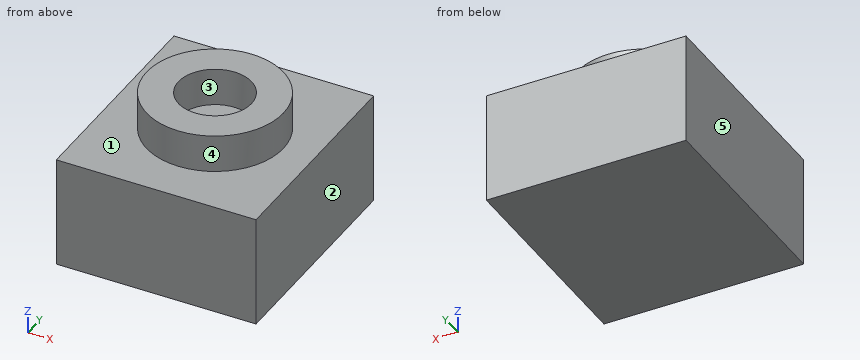
from build123d import *

# Parameters (mm, degrees)
ESQUISSE1_W        = 10.6
ESQUISSE1_H        = 11.7
BOSS_EXTRU_1_DEPTH = 5.9
ESQUISSE2_R        = 3.633546232
ESQUISSE2_R_2      = 1.941835626
BOSS_EXTRU_2_DEPTH = 2


with BuildPart() as part:
    # Esquisse1 → Boss.-Extru.1 (new body)
    with BuildSketch(Plane.XY):
        Rectangle(ESQUISSE1_W, ESQUISSE1_H)
    extrude(amount=BOSS_EXTRU_1_DEPTH)

    # Esquisse2 → Boss.-Extru.2 (add)
    with BuildSketch(Plane.XY.offset(5.9)):
        Circle(ESQUISSE2_R)
        Circle(ESQUISSE2_R_2, mode=Mode.SUBTRACT)
    extrude(amount=BOSS_EXTRU_2_DEPTH)


solid = part.part
Verification items for the finished model (mm, model axes). Face numbers are marked on the shaded views. A direction names the side the tool comes from. Round coordinates to 2 decimals unless told otherwise and drop trailing zeros. Loops run counter-clockwise (first coordinate to the right, second up) from the corner with the lowest first, then second, coordinate; pieces in that order, holes last. Notation, with made-up numbers: (78, -16) - (107, -16) arc R18 ccw to (107, 11) - close; hole circle Ø11 at (2, 32.25). An arc over 180 degrees is marked (long way). Use one line per item in the form item = value.
1. Draft check along X on the marked faces 3, 4 and 5. Enter one of: pulls with the +X half, pulls with the -X half, needs draft (parallel to the pull), parting line crosses it, or undercut.
A:
face_3 = undercut
face_4 = parting line crosses it
face_5 = pulls with the -X half
2. Access from +Z, -Z, +X, -X, +Y, -Y to the whole of each face (thin tool, end or side, straight path). Record for the marked faces 1 and 2.
A:
face_1 = +Z
face_2 = +Z, -Z, +X, +Y, -Y
3. Scan lines: probe 1 along Y at (x, z) = (0, 7.5); probe 2 along Z at (x, y) = (-0.5, -0.25). Record each from-to range of solid material in increasing order.
A:
probe_1 = -3.63 to -1.94, 1.94 to 3.63
probe_2 = 0 to 5.9
4. Section check D-D on y = 4. Record the cut outline in (x, z).
A:
outline = (-5.3, 0) - (5.3, 0) - (5.3, 5.9) - (-5.3, 5.9) - close
5. Section check A-A on x = 0. Record the cut outline in (y, z), and give its area (3 significant figures).
A:
outline = (-5.85, 0) - (5.85, 0) - (5.85, 5.9) - (3.63, 5.9) - (3.63, 7.9) - (1.94, 7.9) - (1.94, 5.9) - (-1.94, 5.9) - (-1.94, 7.9) - (-3.63, 7.9) - (-3.63, 5.9) - (-5.85, 5.9) - close
area = 75.8 mm²
6. Section check B-B on y = 0. Record the cut outline in (x, z).
A:
outline = (-5.3, 0) - (5.3, 0) - (5.3, 5.9) - (3.63, 5.9) - (3.63, 7.9) - (1.94, 7.9) - (1.94, 5.9) - (-1.94, 5.9) - (-1.94, 7.9) - (-3.63, 7.9) - (-3.63, 5.9) - (-5.3, 5.9) - close
7. Section check C-C on z = 7.25. Record the cut outline in (x, y).
A:
outline = circle Ø7.27 at (0, 0); hole circle Ø3.88 at (0, 0)
